Model file for the job. Use its own axes, mm. A direction names the side the tool comes from. Give positions to 0.01 mm unless a question says otherwise; leave off trailing zeros. Write each loop counter-clockwise with the first axis right and the second up, starting at its lowest first coordinate (ties: lowest second). Pieces come first, ordered by that corner, then holes. Notation, with made-up numbers: (-14.75, -15) - (14.25, -15) arc R8 ccw to (14.25, 0) - close; hole circle Ø6 at (17.25, 62.25). An arc over 180 degrees is marked (long way). One line per item, written item: value. Start each with the question number.
(1) Drop flat-ended pins along their axis: P1, Ø1, axis at x = 88, y = 4, coming from the -Z side; P2, Ø4, axis at x = 86.5, z = 20.5, coming from the +Y side; P3, Ø4, axis at y = 8, z = 27, coming from the +X side. Give the stop position or say it passes through.
(2) Cut at D-D, the plane y = 7. List the corners of the cut face in (x, z), and give its area (3 significant figures).
(3) Mould opens along Z. For faces 4 (the face through (98.572, 0.887, 20.071)), 5 (the face through (11, 5, 37)), 6 (the face through (13.88, 5, 25)) say: pulls with the +Z half, pulls with the -Z half, needs draft (parallel to the pull), parting line crosses it, or undercut.
(4) Probe L1, parallel to X at y = 2.5, z = 35; L2, parallel to Z at x = 105, y = 0.7; L3, parallel to Z at x = 31, y = 1.25. List the from-to ranges inside material, lowest first.
(5) Cut at C-C, the plane x = 88. List the corners of the cut face in (y, z), and give its area (3 significant figures).
(6) 3-axis set-ups, long thin cutter, end or side, ignore diameter. For faces 1 (the face through (88, 3, 37)), 2 (the face through (88, 3, 13)), 3 (the face through (90.08, 3, 25)): which of +Z, -Z, +X, -X, +Y, -Y reach the whole face in a straight line?
(7) Cut at A-A, the plane x = 105. List the corners of the cut face in (y, z), and give its area (3 significant figures).
(8) Cut at B-B, the plane z = 25. List the corners of the cut face in (x, y), and give its area (3 significant figures).
from build123d import *

# Parameters (mm, degrees)
SKETCH002_AS_DRAWN_W                      = 5.08
SKETCH002_AS_DRAWN_H                      = 24
EXTRUDE_DEPTH                             = 7.11
EXTRUDE_ONTO_SKETCH002_ROLL_ANGLE         = 90
EXTRUDE_ONTO_SKETCH002_PLACEMENT_ANGLE    = 180
SKETCH003_AS_DRAWN_W                      = 5.08
SKETCH003_AS_DRAWN_H                      = 24
EXTRUDE004_DEPTH                          = 3.3
EXTRUDE004_ONTO_SKETCH003_ROLL_ANGLE      = 90
EXTRUDE004_ONTO_SKETCH003_PLACEMENT_ANGLE = 180
BOX_W                                     = 150
BOX_H                                     = 1.8
BOX_DEPTH                                 = 46
SKETCH_W                                  = 70.612
SKETCH_H                                  = 24.13
POCKET_DEPTH                              = 1.801
SKETCH001_R                               = 8.1
POCKET001_DEPTH                           = 1.801
FILLET_R                                  = 1.5
FILLET001_R                               = 1.5
FILLET002_R                               = 1.5
FILLET003_R                               = 1.5


with BuildPart() as extrude_body:
    # Sketch002 as drawn → Extrude (new)
    with BuildSketch(Plane.XY):
        with Locations((-11.34, 25)):
            Rectangle(SKETCH002_AS_DRAWN_W, SKETCH002_AS_DRAWN_H)
    extrude(amount=EXTRUDE_DEPTH)


with BuildPart() as extrude_body_1:
    # Extrude onto Sketch002 roll: moved
    add(extrude_body.part.rotate(Axis((0, 0, 0), (1, 0, 0)), EXTRUDE_ONTO_SKETCH002_ROLL_ANGLE))


with BuildPart() as extrude_body_2:
    # Extrude onto Sketch002 placement: moved
    add(extrude_body_1.part.moved(Location((0, 1.8, 0))).rotate(Axis((0, 1.8, 0), (0, 0, 1)), EXTRUDE_ONTO_SKETCH002_PLACEMENT_ANGLE))


with BuildPart() as extrude004:
    # Sketch003 as drawn → Extrude004 (new)
    with BuildSketch(Plane.XY):
        with Locations((-87.54, 25)):
            Rectangle(SKETCH003_AS_DRAWN_W, SKETCH003_AS_DRAWN_H)
    extrude(amount=EXTRUDE004_DEPTH)


with BuildPart() as extrude004_1:
    # Extrude004 onto Sketch003 roll: moved
    add(extrude004.part.rotate(Axis((0, 0, 0), (1, 0, 0)), EXTRUDE004_ONTO_SKETCH003_ROLL_ANGLE))


with BuildPart() as extrude004_2:
    # Extrude004 onto Sketch003 placement: moved
    add(extrude004_1.part.moved(Location((0, 1.8, 0))).rotate(Axis((0, 1.8, 0), (0, 0, 1)), EXTRUDE004_ONTO_SKETCH003_PLACEMENT_ANGLE))


with BuildPart() as fusion:
    # Box → Box (new body)
    with BuildSketch(Plane.XY):
        with Locations((75, 0.9)):
            Rectangle(BOX_W, BOX_H)
    extrude(amount=BOX_DEPTH)

    # Sketch → Pocket (cut, through all)
    with BuildSketch(Plane.XZ):
        with Locations((49.323872, 25.120575)):
            Rectangle(SKETCH_W, SKETCH_H)
    extrude(amount=-POCKET_DEPTH, mode=Mode.SUBTRACT)

    # Sketch001 → Pocket001 (cut, through all)
    with BuildSketch(Plane.XZ):
        with Locations((105, 25)):
            Circle(SKETCH001_R)
        with Locations((132, 25)):
            Circle(SKETCH001_R)
    extrude(amount=-POCKET001_DEPTH, mode=Mode.SUBTRACT)

    # Fillet
    fillet_edges = [fusion.edges().sort_by_distance(p)[0] for p in [
        (150, 0.9, 46),
    ]]
    fillet(fillet_edges, radius=FILLET_R)

    # Fillet001
    fillet001_edges = [fusion.edges().sort_by_distance(p)[0] for p in [
        (0, 0.9, 46),
    ]]
    fillet(fillet001_edges, radius=FILLET001_R)

    # Fillet002
    fillet002_edges = [fusion.edges().sort_by_distance(p)[0] for p in [
        (0, 0.9, 0),
    ]]
    fillet(fillet002_edges, radius=FILLET002_R)

    # Fillet003
    fillet003_edges = [fusion.edges().sort_by_distance(p)[0] for p in [
        (150, 0.9, 0),
    ]]
    fillet(fillet003_edges, radius=FILLET003_R)

    # Fusion: union Extrude body, Extrude004
    add(extrude_body_2.part)
    add(extrude004_2.part)


solid = fusion.part
Answers follow:
1. P1: stops at z = 13
1. P2: stops at y = 5.1
1. P3: stops at x = 13.88
2. outline: (8.8, 13) - (13.88, 13) - (13.88, 37) - (8.8, 37) - close
2. area: 122 mm²
3. face 4: undercut
3. face 5: pulls with the +Z half
3. face 6: needs draft
4. L1: x = 8.8 to 13.88, 85 to 90.08
4. L2: z = 0 to 16.9, 33.1 to 46
4. L3: z = 0 to 13.06, 37.19 to 46
5. outline: (0, 0) - (1.8, 0) - (1.8, 13) - (5.1, 13) - (5.1, 37) - (1.8, 37) - (1.8, 46) - (0, 46) - close
5. area: 162 mm²
6. face 1: +Z, +X, -X, +Y
6. face 2: -Z, +X, -X, +Y
6. face 3: +Z, -Z, +X, +Y
7. outline: (0, 0) - (1.8, 0) - (1.8, 16.9) - (0, 16.9) - close; (0, 33.1) - (1.8, 33.1) - (1.8, 46) - (0, 46) - close
7. area: 53.6 mm²
8. outline: (0, 0) - (14.02, 0) - (14.02, 1.8) - (13.88, 1.8) - (13.88, 8.91) - (8.8, 8.91) - (8.8, 1.8) - (0, 1.8) - close; (84.63, 0) - (96.9, 0) - (96.9, 1.8) - (90.08, 1.8) - (90.08, 5.1) - (85, 5.1) - (85, 1.8) - (84.63, 1.8) - close; (113.1, 0) - (123.9, 0) - (123.9, 1.8) - (113.1, 1.8) - close; (140.1, 0) - (150, 0) - (150, 1.8) - (140.1, 1.8) - close
8. area: 137 mm²
